from build123d import *

# Parameters (mm, degrees)
SKETCH1_R                 = 2.75
SKETCH1_R_2               = 1.6
BOSS_EXTRUDE1_DEPTH       = 0.5
SKETCH2_R                 = 4.5
SKETCH2_R_2               = 1.6
BOSS_EXTRUDE2_DEPTH       = 7.4
CHAMFER1_SIZE             = 0.5
SKETCH3_R                 = 4.5
SKETCH3_R_2               = 2.5
BOSS_EXTRUDE3_DEPTH       = 2.2
SKETCH4_R                 = 4.5
SKETCH4_R_2               = 3.05
BOSS_EXTRUDE4_DEPTH       = 2.8
SKETCH5_W                 = 0.8
SKETCH5_H                 = 3.5
CUT_EXTRUDE1_DEPTH        = 4.5
BOSS_EXTRUDE6_START       = -0.5
BOSS_EXTRUDE6_OUTLINE_R   = 4
BOSS_EXTRUDE6_OUTLINE_R_2 = 2.75
BOSS_EXTRUDE6_DEPTH       = 0.5
CUT_EXTRUDE2_START        = -2.2
SKETCH7_R                 = 3.05
CUT_EXTRUDE2_DEPTH        = 2.2


# Read off the part's stored shape, not the designer's step: Boss-Extrude6
with BuildPart() as part:
    # Sketch1 → Boss-Extrude1 (new body)
    with BuildSketch(Plane(origin=(0, 0, 0), x_dir=(0, 1, 0), z_dir=(0, 0, 1))):
        with Locations(Location((0, 0, 0), (0, 0, 270))):
            Circle(SKETCH1_R)
        with Locations(Location((0, 0, 0), (0, 0, 270))):
            Circle(SKETCH1_R_2, mode=Mode.SUBTRACT)
    extrude(amount=BOSS_EXTRUDE1_DEPTH)

    # Sketch2 → Boss-Extrude2 (add)
    with BuildSketch(Plane.XY.offset(0.5)):
        Circle(SKETCH2_R)
        Circle(SKETCH2_R_2, mode=Mode.SUBTRACT)
    extrude(amount=BOSS_EXTRUDE2_DEPTH)

    # Chamfer1
    chamfer1_edges = [part.edges().sort_by_distance(p)[0] for p in [
        (-4.5, 0, 0.5),
    ]]
    chamfer(chamfer1_edges, length=CHAMFER1_SIZE)

    # Sketch3 → Boss-Extrude3 (add)
    with BuildSketch(Plane.XY.offset(7.9)):
        Circle(SKETCH3_R)
        Circle(SKETCH3_R_2, mode=Mode.SUBTRACT)
    extrude(amount=BOSS_EXTRUDE3_DEPTH)

    # Sketch4 → Boss-Extrude4 (add)
    with BuildSketch(Plane.XY.offset(10.1)):
        Circle(SKETCH4_R)
        Circle(SKETCH4_R_2, mode=Mode.SUBTRACT)
    extrude(amount=BOSS_EXTRUDE4_DEPTH)

    # Sketch5 → Cut-Extrude1 (cut, symmetric)
    with BuildSketch(Plane.YZ):
        with Locations((0, 11.15)):
            Rectangle(SKETCH5_W, SKETCH5_H)
    extrude(amount=CUT_EXTRUDE1_DEPTH, both=True, mode=Mode.SUBTRACT)

    # Boss-Extrude6 outline → Boss-Extrude6 (add)
    with BuildSketch(Plane(origin=(0, 0, 0), x_dir=(1, 0, 0), z_dir=(0, 0, -1)).offset(BOSS_EXTRUDE6_START)):
        Circle(BOSS_EXTRUDE6_OUTLINE_R)
        Circle(BOSS_EXTRUDE6_OUTLINE_R_2, mode=Mode.SUBTRACT)
    extrude(amount=BOSS_EXTRUDE6_DEPTH)

    # Sketch7 → Cut-Extrude2 (cut)
    with BuildSketch(Plane.XY.offset(10.1).offset(CUT_EXTRUDE2_START)):
        with Locations(Location((0, 0, 0), (0, 0, 187.535909342))):
            Circle(SKETCH7_R)
    extrude(amount=CUT_EXTRUDE2_DEPTH, mode=Mode.SUBTRACT)


solid = part.part
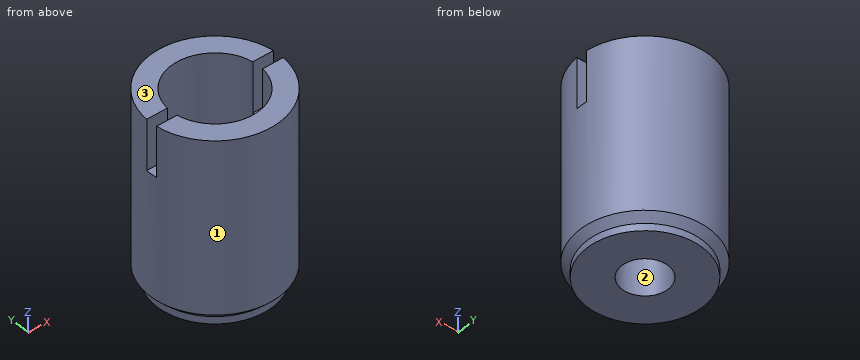
The listing builds one solid part. Answer for the finished solid, in the listing's coordinates (mm). Face numbers are marked on the shaded views. Round coordinates to 2 decimals unless told otherwise and drop trailing zeros. Order: outer loops, then holes, each group sorted by start corner. A loop starts at its lowest first (then second) coordinate and runs counter-clockwise, first axis right, second up. Notation, with made-up numbers: (28, 80.5) -> (68, 80.5) arc R24 cw to (68, 112.5) -> close; hole circle Ø2 at (11, 9.5). An arc over 180 degrees is marked (long way). Put each result on its own line as item: value.
Q1. Section D-D, the plane z = 4.25 is taken. Write down the section's boundary in (x, y).
Results list:
outline: circle Ø9 at (0, 0); hole circle Ø3.2 at (0, 0)
Q2. Each of these flat-tipped pins is pushed along its axis until it touches: P1, Ø3.5, axis at x = 0, y = 0, coming from the +Z side; P2, Ø0.6, axis at x = -4, y = 0, coming from the +Z side; P3, Ø5, axis at y = -3.5, z = 6.5, coming from the +X side. Where does it stop, or does it pass through?
Results list:
P1: z = 7.9
P2: z = 9.4
P3: x = 4.39
Q3. Consider line 1 along Y through (x, z) = (0, 5.25); line 2 along Y through (x, z) = (0, 10.95); line 3 along Z through (x, y) = (-2, -2.25). Determine where each line is inside the solid, lowest interval first.
Results list:
line 1: -4.5 to -1.6, 1.6 to 4.5
line 2: -4.5 to -3.05, 3.05 to 4.5
line 3: 0 to 7.9
Q4. Determine the mould class of the marked faces 1, 2 and 3 for opening direction Y: pulls with the +Y half, pulls with the -Y half, needs draft (parallel to the pull), parting line crosses it, or undercut.
Results list:
face 1: parting line crosses it
face 2: undercut
face 3: needs draft
Q5. Section C-C, the plane y = 0 is taken. Write down the section's boundary in (x, z), and give its area (3 significant figures).
Results list:
outline: (-4.5, 1) -> (-4, 0.5) -> (-4, 0) -> (-1.6, 0) -> (-1.6, 7.9) -> (-3.05, 7.9) -> (-3.05, 9.4) -> (-4.5, 9.4) -> close; (1.6, 0) -> (4, 0) -> (4, 0.5) -> (4.5, 1) -> (4.5, 9.4) -> (3.05, 9.4) -> (3.05, 7.9) -> (1.6, 7.9) -> close
area: 49.4 mm^2
Q6. Section B-B, the plane z = 11.5 is taken. Write down the section's boundary in (x, y).
Results list:
outline: (-4.48, -0.4) arc R4.5 ccw to (4.48, -0.4) -> (3.02, -0.4) arc R3.05 cw to (-3.02, -0.4) -> close; (-4.48, 0.4) -> (-3.02, 0.4) arc R3.05 cw to (3.02, 0.4) -> (4.48, 0.4) arc R4.5 ccw to start
Q7. Section A-A, the plane x = 0 is taken. Write down the section's boundary in (y, z).
Results list:
outline: (-4.5, 1) -> (-4, 0.5) -> (-4, 0) -> (-1.6, 0) -> (-1.6, 7.9) -> (-3.05, 7.9) -> (-3.05, 12.9) -> (-4.5, 12.9) -> close; (1.6, 0) -> (4, 0) -> (4, 0.5) -> (4.5, 1) -> (4.5, 12.9) -> (3.05, 12.9) -> (3.05, 7.9) -> (1.6, 7.9) -> close
